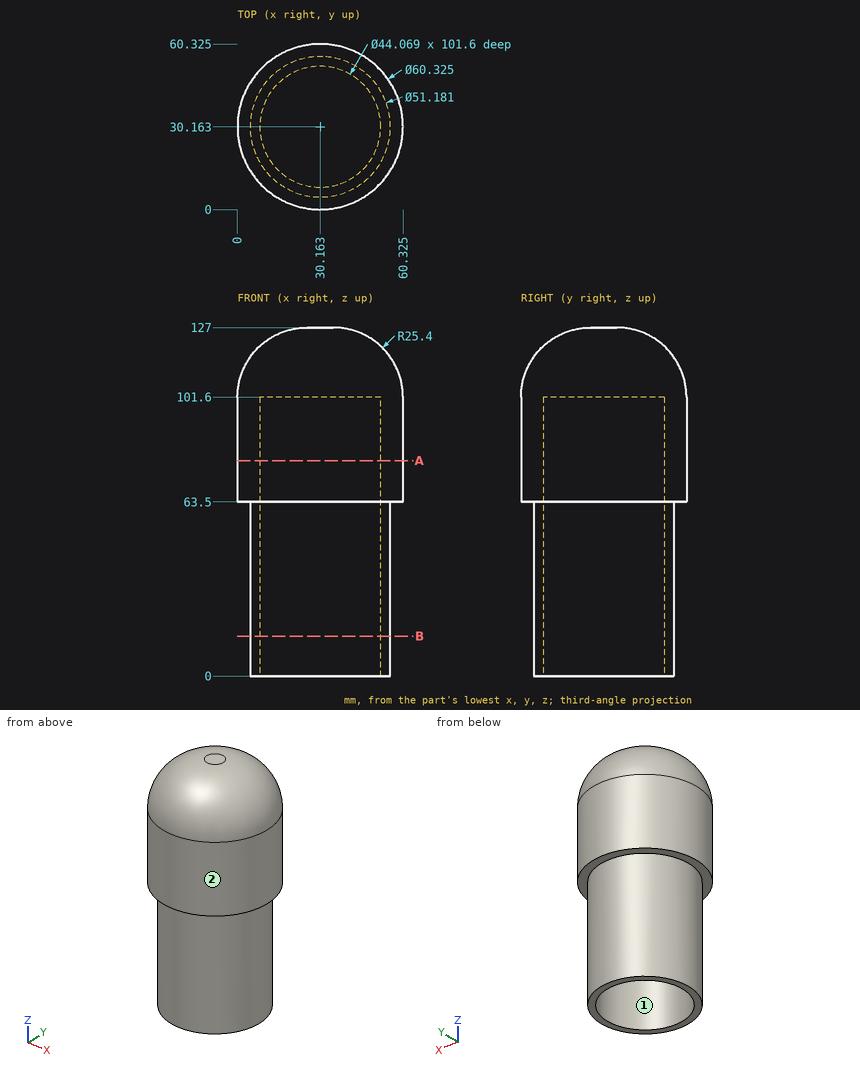
Source: three-view drawing plus pictorial views. Frame: mm from the lowest corner of the part. Round coordinates to 2 decimals unless told otherwise and drop trailing zeros. Loops run counter-clockwise (first coordinate to the right, second up) from the corner with the lowest first, then second, coordinate; pieces in that order, holes last.
1. Section query B-B on z = 14.5. Output: boundary loops of the cut face in (x, y) (1 decimal), and give its area (3 significant figures).
2. Contact query for flat-ended pins moving along their axis: pin 1 (13 mm diameter, centred on x = 28, y = 30, fed in from -Z); pin 2 (1.5 mm diameter, centred on y = 41.5, z = 103, fed in from +X); pin 3 (6 mm diameter, centred on x = 52, y = 27, fed in from +Z). Output: stop coordinate, or through.
3. Section query A-A on z = 78.5. Output: boundary loops of the cut face in (x, y) (1 decimal).
4. Mould query, pull axis X, two halves, no side actions, for the marked faces 1 and 2. Classes: released by +X, released by -X, zero draft, split by the parting line, or undercut.
5. Ray query, L1, parallel to X at y = 12, z = 26.5 (1 decimal); L2, parallel to X at y = 49.5, z = 38.5 (1 decimal); L3, parallel to Y at x = 36, z = 27 (1 decimal). Return the intervals inside material, ascending.
Answers below:
1. outline: circle Ø51.2 at (30.2, 30.2); hole circle Ø44.1 at (30.2, 30.2)
1. area: 532 mm2
2. pin 1: stops at z = 101.6
2. pin 2: stops at x = 58.37
2. pin 3: stops at z = 122.59
3. outline: circle Ø60.3 at (30.2, 30.2); hole circle Ø44.1 at (30.2, 30.2)
4. face 1: undercut
4. face 2: split by the parting line
5. L1: x = 12.1 to 17.7, 42.6 to 48.2
5. L2: x = 13.4 to 19.6, 40.7 to 46.9
5. L3: y = 5.2 to 8.9, 51.4 to 55.1
